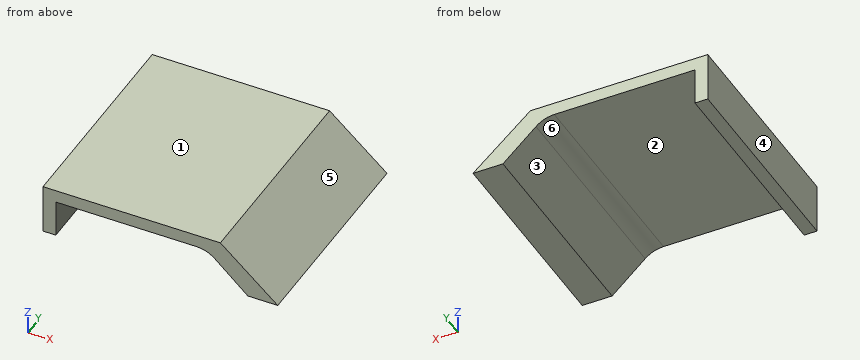
from build123d import *

# Parameters (mm, degrees)
F1_DEPTH = 50


with BuildPart() as f1:
    # F0 (on Front) → F1 (new body)
    with BuildSketch(Plane.XZ):
        with BuildLine():
            Line((-20.327587, 11.793104), (-20.327587, 0))
            Line((-20.327587, 0), (-17.327587, 0))
            Line((-17.327587, 0), (-17.327587, 8.793104))
            Line((-17.327587, 8.793104), (15.628933, 8.793104))
            ThreePointArc((15.628933, 8.793104), (17.934571, 8.359736), (19.925504, 7.118783))
            Line((19.925504, 7.118783), (27.672413, 0))
            Line((27.672413, 0), (34.672413, 0))
            Line((34.672413, 0), (21.224136, 11.793104))
            Line((21.224136, 11.793104), (-20.327587, 11.793104))
        make_face()
    extrude(amount=F1_DEPTH)


solid = f1.part
The listing builds one solid part. Answer for the finished solid, in the listing's coordinates (mm). Face numbers are marked on the shaded views. A direction names the side the tool comes from. Coordinates: 2 decimals unless noted, no trailing zeros. Order: outer loops, then holes, each group sorted by start corner. A loop starts at its lowest first (then second) coordinate and runs counter-clockwise, first axis right, second up. Notation, with made-up numbers: (-26.5, 81) -> (27.5, 81) arc R17 ccw to (27.5, 103) -> close; hole circle Ø1 at (18.25, -19.5). An arc over 180 degrees is marked (long way). Answer in a Markdown table with one row per item. Add a question column.
Item 1: Which of the six approach directions +Z, -Z, +X, -X, +Y, -Y give full straight-line access (tool end or side, diameter ignored) to the marked faces 5 and 6?
Item 2: Find section D-D (z = 2.75). Write down the section's boundary in (x, y).
Item 3: Find section A-A (z = 6). Write down the section's boundary in (x, y), then the cut area to 3 significant figures.
Item 4: Each of these flat-tipped pins is pushed along its axis until it touches: P1, Ø8, axis at x = -13, y = -43, coming from the -Z side; P2, Ø3, axis at x = 18, z = 5, coming from the -Y side; P3, Ø7, axis at y = -31.5, z = 5.5, coming from the +X side; P4, Ø4, axis at x = 23.5, z = 6, coming from the +Y side. Where does it stop, or does it pass through?
Item 5: Determine the mould class of the marked faces 1, 2, 3 and 4 for opening direction X: +X half, -X half, draft (parallel to the pull), parting line (faces both ways), or undercut.
Item 6: Find the intervals of material crossed by L1, parallel to Z at x = -1, y = -15.5; L2, parallel to X at y = -26.5, z = 0.75; L3, parallel to X at y = -27, z = 7, in increasing order. Write a range as from..to.
Item 7: Find section B-B (y = -29.5). Write down the section's boundary in (x, z), then the cut area to 3 significant figures.
Item 8: Find section C-C (x = 14). Write down the section's boundary in (y, z).
Result set:
| question | item | result |
|---|---|---|
| 1 | face 5 | +Z, +X, +Y, -Y |
| 1 | face 6 | -Z, +Y, -Y |
| 2 | outline | (-20.33, -50) -> (-17.33, -50) -> (-17.33, 0) -> (-20.33, 0) -> close; (24.68, -50) -> (31.54, -50) -> (31.54, 0) -> (24.68, 0) -> close |
| 3 | outline | (-20.33, -50) -> (-17.33, -50) -> (-17.33, 0) -> (-20.33, 0) -> close; (21.14, -50) -> (27.83, -50) -> (27.83, 0) -> (21.14, 0) -> close |
| 3 | area | 484 mm² |
| 4 | P1 | stops at z = 8.79 |
| 4 | P2 | passes through |
| 4 | P3 | stops at x = 32.39 |
| 4 | P4 | stops at y = 0 |
| 5 | face 1 | draft |
| 5 | face 2 | undercut |
| 5 | face 3 | undercut |
| 5 | face 4 | -X half |
| 6 | L1 | z = 8.79..11.79 |
| 6 | L2 | x = -20.33..-17.33, 26.86..33.82 |
| 6 | L3 | x = -20.33..-17.33, 20.05..26.69 |
| 7 | outline | (-20.33, 0) -> (-17.33, 0) -> (-17.33, 8.79) -> (15.63, 8.79) arc R6.35 cw to (19.93, 7.12) -> (27.67, 0) -> (34.67, 0) -> (21.22, 11.79) -> (-20.33, 11.79) -> close |
| 7 | area | 216 mm² |
| 8 | outline | (-50, 8.79) -> (0, 8.79) -> (0, 11.79) -> (-50, 11.79) -> close |
